Here's the drawing with two shaded views (mm, measured from the low corner). I have some questions. Give positions to 0.01 mm unless a question says otherwise; leave off trailing zeros. Write each loop counter-clockwise with the first axis right and the second up, starting at its lowest first coordinate (ties: lowest second). Pieces come first, ordered by that corner, then holes. Notation, with made-up numbers: (70, -18.75) - (84, -18.75) arc R20 cw to (84, 9.25) - close; hole circle Ø2 at (-9.75, 15). An arc over 180 degrees is marked (long way). Write item = value, one per line.
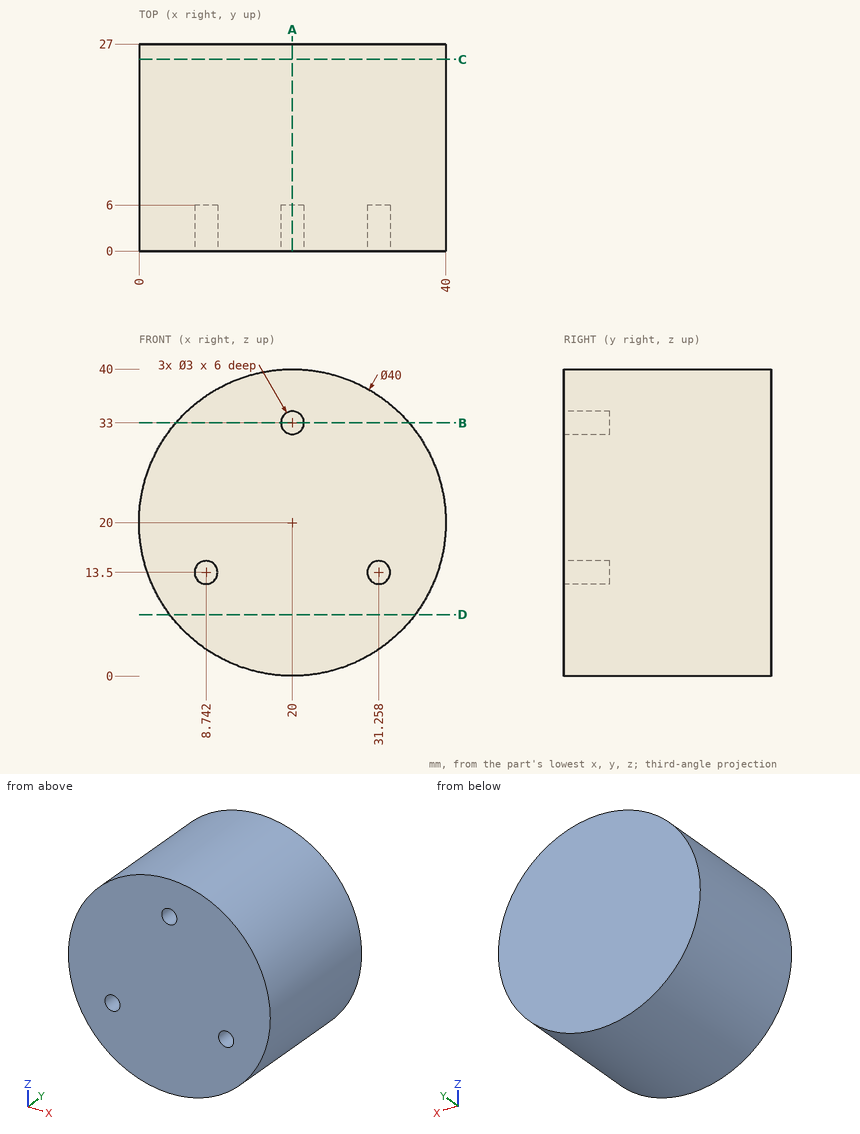
1. If we section it at B-B, the plane z = 33: Please give me the cut outline in (x, y).
Filled sheet:
outline = (4.8, 0) - (18.5, 0) - (18.5, 6) - (21.5, 6) - (21.5, 0) - (35.2, 0) - (35.2, 27) - (4.8, 27) - close
2. If we section it at D-D, the plane z = 8: Please give me the cut outline in (x, y).
Filled sheet:
outline = (4, 0) - (36, 0) - (36, 27) - (4, 27) - close
3. If we section it at A-A, the plane x = 20: Please give me the cut outline in (y, z), and give its area (3 significant figures).
Filled sheet:
outline = (0, 0) - (27, 0) - (27, 40) - (0, 40) - (0, 34.5) - (6, 34.5) - (6, 31.5) - (0, 31.5) - close
area = 1,060 mm2
4. For pin 1 (2.5 mm diameter, centred on x = 20, z = 33, fed in from -Y); pin 2 (1.5 mm diameter, centred on y = 19.5, z = 25.5, fed in from +X); pin 3 (3 mm diameter, centred on y = 8.5, z = 6, fed in from +X), each with a flat end and sliding along its axis, tell me the tip position at first contact or that it passes through.
Filled sheet:
pin_1 = 6
pin_2 = 39.43
pin_3 = 35.61
5. If we section it at C-C, the plane y = 25: Please give me the cut outline in (x, z).
Filled sheet:
outline = circle Ø40 at (20, 20)
6. I need wall thicknesses on line 1 (X direction, y = 1.3, z = 13.5) (1 decimal); line 2 (X direction, y = 4, z = 13) (1 decimal); line 3 (X direction, y = 4.65, z = 33). Which ranges of each line are inside material? Lowest first, please.
Filled sheet:
line_1 = 1.1 to 7.2, 10.2 to 29.8, 32.8 to 38.9
line_2 = 1.3 to 7.3, 10.2 to 29.8, 32.7 to 38.7
line_3 = 4.8 to 18.5, 21.5 to 35.2
